Autodesk Inventor part; units mm, degrees
ref_plane "YZ Plane" through (0, 0, 0) normal (1, 0, 0) x (0, 1, 0)
ref_plane "XZ Plane" through (0, 0, 0) normal (0, 1, 0) x (-1, 0, 0)
ref_plane "XY Plane" through (0, 0, 0) normal (0, 0, 1) x (1, 0, 0)
sketch "Sketch1" plane through (0, 0, 0) normal (0, 0, 1) x (1, 0, 0)
  line L0 (0, 0) -> (0, 40)
  line L1 (0, 40) -> (50, 40)
  line L2 (50, 40) -> (50, 36)
  line L3 (50, 36) -> (7, 36)
  line L4 (7, 36) -> (7, 0)
  line L5 (7, 0) -> (0, 0)
  dimension "d0" = 40
  dimension "d1" = 43
  dimension "d2" = 4
  dimension "d3" = 7
extrude "Extrusion1" add sketch "Sketch1" along normal blind 43
sketch "Sketch2" plane through (0, 0, 43) normal (0, 0, 1) x (1, 0, 0)
  line L0 (7, 0) -> (7, 36)
  line L1 (7, 36) -> (50, 36)
  line L2 (50, 36) -> (50, 40)
  line L3 (50, 40) -> (0, 40)
  line L4 (0, 40) -> (0, 0)
  line L5 (0, 0) -> (7, 0)
  line L6 (7, 0) -> (7, 36)
  line L7 (7, 36) -> (50, 36)
  line L8 (7, 0) -> (50, 36)
extrude "Extrusion2" add sketch "Sketch2" along normal blind 2
sketch "Sketch3" plane through (0, 0, 0) normal (0, 0, -1) x (-1, 0, 0)
  line L0 (-7, 0) -> (-7, 36)
  line L1 (0, 0) -> (-7, 0)
  line L2 (0, 40) -> (0, 0)
  line L3 (-50, 40) -> (0, 40)
  line L4 (-50, 36) -> (-50, 40)
  line L5 (-7, 36) -> (-50, 36)
  line L6 (0, 0) -> (-7, 0)
  line L7 (-7, 0) -> (-50, 36)
  line L8 (-7, 0) -> (-50, 36)
extrude "Extrusion3" add sketch "Sketch3" along normal blind 2
sketch "Sketch4" plane through (7, 36, 43) normal (0, -1, 0) x (1, 0, 0)
  line L0 (0, -43) -> (43, -43)
  line L1 (43, -43) -> (43, 0)
  line L2 (0, 0) -> (43, 0)
  line L3 (0, -43) -> (0, 0)
  line L4 (37, -6) -> (6, -6) construction
  line L5 (6, -6) -> (6, -37) construction
  line L6 (6, -37) -> (37, -37) construction
  line L7 (37, -37) -> (37, -6) construction
  line L8 (0, 0) -> (43, 0) construction
  point P0 (-7, -43)
  point P1 (21.5, -21.5)
  point P2 (37, -21.5)
  point P3 (43, -21.5)
  point P4 (21.5, 0)
  point P5 (21.5, -6)
  dimension "d10" = 31
  dimension "d11" = 31
hole "Hole1" at (44, 36, 37) at (44, 36, 6) at (13, 36, 6) at (13, 36, 37) direction (0, 1, 0) diameter 3.2 end through all
hole "Hole2" at (28.5, 36, 21.5) direction (0, 1, 0) diameter 25 end through all
sketch "Sketch5" plane through (0, 0, 45) normal (-1, 0, 0) x (0, 0, 1)
  line L0 (-47, 40) -> (0, 40)
  line L1 (-47, 0) -> (0, 0)
  point P0 (-45, 0)
  point P1 (-23.5, 30)
  point P2 (-23.5, 10)
  point P3 (-23.5, 40)
  dimension "d26" = 10
  dimension "d27" = 10
hole "Hole3" at (0, 30, 21.5) at (0, 10, 21.5) direction (1, 0, 0) diameter 5.2 end through all
sketch "Sketch6" plane through (7, 0, 43) normal (1, 0, 0) x (0, 0, -1)
  circle A0 centre (21.5, 30) radius 2.6
  circle A1 centre (21.5, 10) radius 2.6
  line L0 (43, 0) -> (43, 36)
  line L1 (43, 36) -> (0, 36)
  line L2 (0, 0) -> (0, 36)
  line L3 (43, 0) -> (0, 0)
  circle A2 centre (21.5, 30) radius 5
  circle A3 centre (21.5, 10) radius 5
  point P0 (43, 0)
  dimension "d35" = 10
  dimension "d36" = 10
extrude "Extrusion4" cut sketch "Sketch6" against normal blind 3 contours A2 | A3
properties part number "Extruder Mount"
Geometry check sheet. Reference: the model listing, model coordinates, mm. A direction names the side the tool comes from. Round coordinates to 2 decimals unless told otherwise and drop trailing zeros. Order: outer loops, then holes, each group sorted by start corner. A loop starts at its lowest first (then second) coordinate and runs counter-clockwise, first axis right, second up. Notation, with made-up numbers: (-40, -3) - (-7, -3) arc R13 cw to (-7, 7) - close; hole circle Ø9 at (76.5, 14.5). An arc over 180 degrees is marked (long way). Use a Markdown table: item, result. Add a question column.
(1) Sectioned sample at A-A, the plane z = 37. Enter the section's corners in (x, y), and give its area (3 significant figures).
(2) Sectioned sample at D-D, the plane y = 29. Enter the section's corners in (x, z), and give its area (3 significant figures).
(3) Sectioned sample at C-C, the plane x = 28.5. Enter the section's corners in (y, z), and give its area (3 significant figures).
(4) Sectioned sample at B-B, the plane z = 21.5. Enter the section's corners in (x, y).
(5) Tool access check on faces 1 (the flat face through (19, 26, 0)), 2 (the cylindrical face through (36.106, 38.028, 31.42)), 3 (the cylindrical face through (5.521, 13.379, 25.185)). Record the directions out of +Z, -Z, +X, -X, +Y, -Y that give a thin tool (end or side, any length) a straight path to the whole face; none if there is none.
(6) Material ranges on line 1 along Y through (x, z) = (2.6, 21.5); line 2 along Y through (x, z) = (5.95, 21.5); line 3 along Z through (x, y) = (44, 38.4), recorded low to high. Write a range as [from, to].
(7) Depth check by flat-ended pin: pin 1 (1.5 mm diameter, centred on x = 10, z = 27.5, fed in from -Y); pin 2 (11 mm diameter, centred on y = 28.5, z = 20, fed in from +X). Enter the tip coordinate at first touch or a pass-through.
(8) Release check for a two-part mould opening along Z. For faces 4 (the flat face through (19, 25, 45)), 5 (the flat face through (4, 28, 19)), 6 (the cylindrical face through (2.028, 12.307, 22.7)), 7 (the flat face through (50, 38, 21)) record: pulls with the +Z half, pulls with the -Z half, needs draft (parallel to the pull), parting line crosses it, or undercut.
Answers below:
| question | item | result |
|---|---|---|
| 1 | outline | (0, 0) - (7, 0) - (7, 36) - (11.4, 36) - (11.4, 40) - (0, 40) - close; (14.6, 36) - (42.4, 36) - (42.4, 40) - (14.6, 40) - close; (45.6, 36) - (50, 36) - (50, 40) - (45.6, 40) - close |
| 1 | area | 426 mm² |
| 2 | outline | (0, -2) - (41.64, -2) - (41.64, 0) - (7, 0) - (7, 16.6) - (4, 16.6) - (4, 19.1) - (0, 19.1) - close; (0, 23.9) - (4, 23.9) - (4, 26.4) - (7, 26.4) - (7, 43) - (41.64, 43) - (41.64, 45) - (0, 45) - close |
| 2 | area | 419 mm² |
| 3 | outline | (18, -2) - (40, -2) - (40, 9) - (36, 9) - (36, 0) - (18, 0) - close; (18, 43) - (36, 43) - (36, 34) - (40, 34) - (40, 45) - (18, 45) - close |
| 3 | area | 160 mm² |
| 4 | outline | (0, 0) - (7, 0) - (7, 5) - (4, 5) - (4, 7.4) - (0, 7.4) - close; (0, 12.6) - (4, 12.6) - (4, 15) - (7, 15) - (7, 25) - (4, 25) - (4, 27.4) - (0, 27.4) - close; (0, 32.6) - (4, 32.6) - (4, 35) - (7, 35) - (7, 36) - (16, 36) - (16, 40) - (0, 40) - close; (41, 36) - (50, 36) - (50, 40) - (41, 40) - close |
| 5 | face 1 | +X, -Y |
| 5 | face 2 | +Y, -Y |
| 5 | face 3 | +X |
| 6 | line 1 | [0, 7.4], [12.6, 27.4], [32.6, 40] |
| 6 | line 2 | [0, 5], [15, 25], [35, 40] |
| 6 | line 3 | [-2, 4.4], [7.6, 35.4], [38.6, 45] |
| 7 | pin 1 | y = 36 |
| 7 | pin 2 | x = 7 |
| 8 | face 4 | pulls with the +Z half |
| 8 | face 5 | undercut |
| 8 | face 6 | undercut |
| 8 | face 7 | needs draft |
